Part model, mm, in its own coordinate system. Face numbers are marked on the shaded views. A direction names the side the tool comes from. Give positions to 0.01 mm unless a question says otherwise; leave off trailing zeros. Order: outer loops, then holes, each group sorted by start corner. A loop starts at its lowest first (then second) coordinate and runs counter-clockwise, first axis right, second up. Notation, with made-up numbers: (-27.5, 59) - (12.5, 59) arc R26 cw to (12.5, 84) - close; hole circle Ø4 at (35, 28.25). An arc over 180 degrees is marked (long way). One line per item, written item: value.
```python
from build123d import *

# Parameters (mm, degrees)
CROQUIS1_R              = 2.1
SALIENTE_EXTRUIR1_DEPTH = 5
CROQUIS2_W              = 71.4
CROQUIS2_H              = 20
CROQUIS2_R              = 2.1
SALIENTE_EXTRUIR2_DEPTH = 5
CORTAR_EXTRUIR1_REACH   = 83.994
CROQUIS4_R              = 1
CORTAR_EXTRUIR2_START   = -5
CROQUIS5_R              = 2.1
CORTAR_EXTRUIR2_DEPTH   = 3


with BuildPart() as part:
    # Croquis1 → Saliente-Extruir1 (new body)
    with BuildSketch(Plane.XY):
        Polygon((26, 20), (-4, 20), (-4, -4), (4, -4), (4, 0), (26, 0), align=None)
        Circle(CROQUIS1_R, mode=Mode.SUBTRACT)
    extrude(amount=SALIENTE_EXTRUIR1_DEPTH)

    # Croquis2 → Saliente-Extruir2 (add)
    with BuildSketch(Plane(origin=(26, 0, 0), x_dir=(0, 0, -1), z_dir=(1, 0, 0))):
        with Locations((-35.7, 10)):
            Rectangle(CROQUIS2_W, CROQUIS2_H)
        with Locations((-49.4, 10)):
            Circle(CROQUIS2_R, mode=Mode.SUBTRACT)
    extrude(amount=SALIENTE_EXTRUIR2_DEPTH)

    # Croquis4 → Cortar-Extruir1 (cut, up to next)
    with BuildSketch(Plane(origin=(31, 0, 0), x_dir=(0, 0, -1), z_dir=(1, 0, 0)), mode=Mode.PRIVATE) as cortar_extruir1_sk1:
        with Locations((-68.4, 10)):
            Circle(CROQUIS4_R)
    cortar_extruir1_tool1 = extrude(cortar_extruir1_sk1.sketch, amount=-CORTAR_EXTRUIR1_REACH, mode=Mode.PRIVATE) & part.part
    # Croquis4 → Cortar-Extruir1 (cut, up to next)
    with BuildSketch(Plane(origin=(31, 0, 0), x_dir=(0, 0, -1), z_dir=(1, 0, 0)), mode=Mode.PRIVATE) as cortar_extruir1_sk2:
        with Locations((-64.9, 10)):
            Circle(CROQUIS4_R)
    cortar_extruir1_tool2 = extrude(cortar_extruir1_sk2.sketch, amount=-CORTAR_EXTRUIR1_REACH, mode=Mode.PRIVATE) & part.part
    # Croquis4 → Cortar-Extruir1 (cut, up to next)
    with BuildSketch(Plane(origin=(31, 0, 0), x_dir=(0, 0, -1), z_dir=(1, 0, 0)), mode=Mode.PRIVATE) as cortar_extruir1_sk3:
        with Locations((-61.4, 10)):
            Circle(CROQUIS4_R)
    cortar_extruir1_tool3 = extrude(cortar_extruir1_sk3.sketch, amount=-CORTAR_EXTRUIR1_REACH, mode=Mode.PRIVATE) & part.part
    # Croquis4 → Cortar-Extruir1 (cut, up to next)
    with BuildSketch(Plane(origin=(31, 0, 0), x_dir=(0, 0, -1), z_dir=(1, 0, 0)), mode=Mode.PRIVATE) as cortar_extruir1_sk4:
        with Locations((-57.9, 10)):
            Circle(CROQUIS4_R)
    cortar_extruir1_tool4 = extrude(cortar_extruir1_sk4.sketch, amount=-CORTAR_EXTRUIR1_REACH, mode=Mode.PRIVATE) & part.part
    # Croquis4 → Cortar-Extruir1 (cut, up to next)
    with BuildSketch(Plane(origin=(31, 0, 0), x_dir=(0, 0, -1), z_dir=(1, 0, 0)), mode=Mode.PRIVATE) as cortar_extruir1_sk5:
        with Locations((-40.9, 10)):
            Circle(CROQUIS4_R)
    cortar_extruir1_tool5 = extrude(cortar_extruir1_sk5.sketch, amount=-CORTAR_EXTRUIR1_REACH, mode=Mode.PRIVATE) & part.part
    # Croquis4 → Cortar-Extruir1 (cut, up to next)
    with BuildSketch(Plane(origin=(31, 0, 0), x_dir=(0, 0, -1), z_dir=(1, 0, 0)), mode=Mode.PRIVATE) as cortar_extruir1_sk6:
        with Locations((-37.4, 10)):
            Circle(CROQUIS4_R)
    cortar_extruir1_tool6 = extrude(cortar_extruir1_sk6.sketch, amount=-CORTAR_EXTRUIR1_REACH, mode=Mode.PRIVATE) & part.part
    # Croquis4 → Cortar-Extruir1 (cut, up to next)
    with BuildSketch(Plane(origin=(31, 0, 0), x_dir=(0, 0, -1), z_dir=(1, 0, 0)), mode=Mode.PRIVATE) as cortar_extruir1_sk7:
        with Locations((-33.9, 10)):
            Circle(CROQUIS4_R)
    cortar_extruir1_tool7 = extrude(cortar_extruir1_sk7.sketch, amount=-CORTAR_EXTRUIR1_REACH, mode=Mode.PRIVATE) & part.part
    # Croquis4 → Cortar-Extruir1 (cut, up to next)
    with BuildSketch(Plane(origin=(31, 0, 0), x_dir=(0, 0, -1), z_dir=(1, 0, 0)), mode=Mode.PRIVATE) as cortar_extruir1_sk8:
        with Locations((-30.4, 10)):
            Circle(CROQUIS4_R)
    cortar_extruir1_tool8 = extrude(cortar_extruir1_sk8.sketch, amount=-CORTAR_EXTRUIR1_REACH, mode=Mode.PRIVATE) & part.part
    add(cortar_extruir1_tool1.solids().sort_by_distance((31, 10, 68.4))[0], mode=Mode.SUBTRACT)
    add(cortar_extruir1_tool2.solids().sort_by_distance((31, 10, 64.9))[0], mode=Mode.SUBTRACT)
    add(cortar_extruir1_tool3.solids().sort_by_distance((31, 10, 61.4))[0], mode=Mode.SUBTRACT)
    add(cortar_extruir1_tool4.solids().sort_by_distance((31, 10, 57.9))[0], mode=Mode.SUBTRACT)
    add(cortar_extruir1_tool5.solids().sort_by_distance((31, 10, 40.9))[0], mode=Mode.SUBTRACT)
    add(cortar_extruir1_tool6.solids().sort_by_distance((31, 10, 37.4))[0], mode=Mode.SUBTRACT)
    add(cortar_extruir1_tool7.solids().sort_by_distance((31, 10, 33.9))[0], mode=Mode.SUBTRACT)
    add(cortar_extruir1_tool8.solids().sort_by_distance((31, 10, 30.4))[0], mode=Mode.SUBTRACT)

    # Croquis5 → Cortar-Extruir2 (cut)
    with BuildSketch(Plane(origin=(31, 0, 0), x_dir=(0, 0, -1), z_dir=(1, 0, 0)).offset(CORTAR_EXTRUIR2_START)):
        with Locations((-57.9, 10)):
            Circle(CROQUIS5_R)
        with Locations((-64.9, 10)):
            Circle(CROQUIS5_R)
        with Locations((-40.9, 10)):
            Circle(CROQUIS5_R)
        with Locations((-33.9, 10)):
            Circle(CROQUIS5_R)
    extrude(amount=CORTAR_EXTRUIR2_DEPTH, mode=Mode.SUBTRACT)


solid = part.part
```
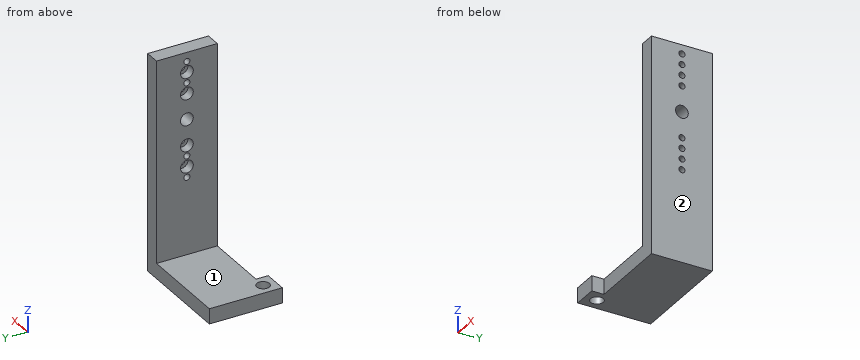
1) Cut at C-C, the plane z = 33.9. Give the cut face in (x, y), then the cut area to 3 significant figures.
Outcome:
outline: (26, 0) - (31, 0) - (31, 9) - (29, 9) - (29, 7.9) - (26, 7.9) - close; (26, 12.1) - (29, 12.1) - (29, 11) - (31, 11) - (31, 20) - (26, 20) - close
area: 83.4 mm^2
2) Which spindle directions (+Z, -Z, +X, -X, +Y, -Y) get a long thin tool onto all of the face, cutting with end or side? Do the marked faces 1 and 2. Say none if no direction does.
Outcome:
face 1: +Z, -X, +Y, -Y
face 2: +Z, -Z, +X, +Y, -Y
3) Cut at A-A, the plane z = 61.4. Give the cut face in (x, y).
Outcome:
outline: (26, 0) - (31, 0) - (31, 9) - (26, 9) - close; (26, 11) - (31, 11) - (31, 20) - (26, 20) - close
4) Cut at B-B, the plane x = 0. Give the cut face in (y, z), then the cut area to 3 significant figures.
Outcome:
outline: (-4, 0) - (-2.1, 0) - (-2.1, 5) - (-4, 5) - close; (2.1, 0) - (20, 0) - (20, 5) - (2.1, 5) - close
area: 99.0 mm^2
5) Drill centre lines: line 1 along X through (y, z) = (3, 46); line 2 along Z through (x, y) = (5.5, 19); line 3 along Y through (x, z) = (28, 68). Where is each one in solid material? Low to high. Write a range as from..to.
Outcome:
line 1: x = 26..31
line 2: z = 0..5
line 3: y = 0..9.08, 10.92..20
6) Pin check, flat tips, straight feed: pin 1 (4.5 mm diameter, centred on y = 11, z = 34.5, fed in from -X); pin 2 (5 mm diameter, centred on y = 10, z = 33.9, fed in from +X); pin 3 (1.3 mm diameter, centred on y = 10.5, z = 40, fed in from -X); pin 4 (12 mm diameter, centred on x = 15.5, y = 3.5, fed in from +Z). Stop position of each tip, or through.
Outcome:
pin 1: stops at x = 26
pin 2: stops at x = 31
pin 3: stops at x = 29
pin 4: stops at z = 5
7) Cut at D-D, the plane y = 15. Give the cut face in (x, z), then the cut area to 3 significant figures.
Outcome:
outline: (-4, 0) - (31, 0) - (31, 71.4) - (26, 71.4) - (26, 5) - (-4, 5) - close
area: 507 mm^2
